```python
from build123d import *

# Parameters (mm, degrees)
SKETCH1_W           = 10.000000000000004
SKETCH1_H           = 10
SKETCH1_W_2         = 10
BOSS_EXTRUDE1_DEPTH = 60
CHAMFER1_SIZE       = 3
SKETCH2_R           = 2.5
BOSS_EXTRUDE2_DEPTH = 5
BOSS_EXTRUDE3_START = -65
SKETCH2_2_R         = 2.5
BOSS_EXTRUDE3_DEPTH = 5
CHAMFER2_SIZE       = 1
CHAMFER2_SIZE2      = 1.6731571851015
CHAMFER3_SIZE       = 0.75


with BuildPart() as part:
    # Sketch1 → Boss-Extrude1 (new body)
    with BuildSketch(Plane.XY):
        with Locations((-27.101007166283644, 56.98463103929536)):
            Rectangle(SKETCH1_W, SKETCH1_H)
        Polygon((-12.10100716628364, 51.98463103929536), (-15.740709508945711, 61.98463103929536), (-22.10100716628364, 61.98463103929536), (-22.10100716628364, 51.98463103929536), (-5, 5), (5, 5), align=None)
        Rectangle(SKETCH1_W_2, SKETCH1_H)
    extrude(amount=BOSS_EXTRUDE1_DEPTH)

    # Chamfer1
    chamfer1_edges = [part.edges().sort_by_distance(p)[0] for p in [
        (-5, -5, 30),
    ]]
    chamfer(chamfer1_edges, length=CHAMFER1_SIZE)

    # Sketch2 → Boss-Extrude2 (add)
    with BuildSketch(Plane.XY.offset(60)):
        Circle(SKETCH2_R)
    extrude(amount=BOSS_EXTRUDE2_DEPTH)

    # Sketch2<2> → Boss-Extrude3 (add)
    with BuildSketch(Plane.XY.offset(60).offset(BOSS_EXTRUDE3_START)):
        Circle(SKETCH2_2_R)
    extrude(amount=BOSS_EXTRUDE3_DEPTH)

    # Chamfer2
    chamfer2_edges = [part.edges().sort_by_distance(p)[0] for p in [
        (-15.740709508945711, 61.98463103929536, 30),
    ]]
    chamfer2_side = [part.faces().sort_by_distance(p)[0] for p in [
        (-5.3703547544728565, 33.492315519647676, 30),
    ]]
    chamfer(chamfer2_edges, length=CHAMFER2_SIZE, length2=CHAMFER2_SIZE2, reference=chamfer2_side[0])

    # Chamfer3
    chamfer3_edges = [part.edges().sort_by_distance(p)[0] for p in [
        (-2.5, 3.1e-16, 65),
        (-2.5, 3.1e-16, -5),
    ]]
    chamfer(chamfer3_edges, length=CHAMFER3_SIZE)


solid = part.part
```
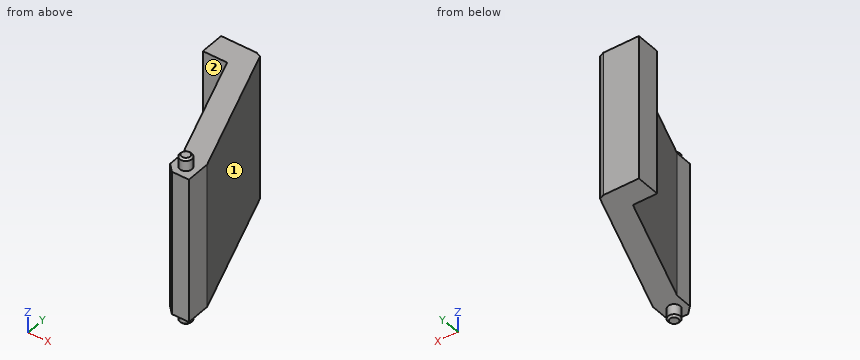
For this review, take the finished solid that the model builds, in its own axes (mm). Face numbers are marked on the shaded views. A direction names the side the tool comes from. Round coordinates to 2 decimals unless told otherwise and drop trailing zeros. Write each loop counter-clockwise with the first axis right and the second up, starting at its lowest first coordinate (ties: lowest second). Pieces come first, ordered by that corner, then holes. Notation, with made-up numbers: (27, 1) - (81, 1) arc R9 cw to (81, 15) - close; hole circle Ø3 at (31.5, 63.25). An arc over 180 degrees is marked (long way). Answer as CSV lines item,"result". Start each with the question number.
(1) Add section D-D, the plane x = -25. State the section outline as (y, z) points, plus the area to 3 significant figures.
(2) For line 1 (Y direction, x = -24, z = 32.5); line 2 (X direction, y = -1, z = 2.5); line 3 (Z direction, x = -7.5, y = 36), list the stretches that pass through material, from the lowest coordinate up.
(3) Machinability: for the marked faces 1 and 2, which of the approach directions +Z, -Z, +X, -X, +Y, -Y give a long, thin tool a straight path to every point of the face, cutting with its end or side? Answer none if there is none.
(4) For pin 1 (7.5 mm diameter, centred on y = 1.5, z = 24, fed in from -X); pin 2 (18.5 mm diameter, centred on x = -7, y = 30.5, fed in from -Z); pin 3 (3 mm diameter, centred on y = 33, z = 22.5, fed in from +X); pin 4 (5 mm diameter, centred on x = -11.5, y = 11.5, fed in from +Z), all flat-tipped, find the tip position at first contact; note any pin that passes through.
(5) Add section C-C, the plane x = 0. State the section outline as (y, z) points, plus the area to 3 significant figures.
(6) Add section B-B, the plane y = 0. State the section outline as (x, z) points, plus the area to 3 significant figures.
(7) Add section A-A, the plane z = 32. State the section outline as (x, y) points, plus the area to 3 significant figures.
From the geometry:
1,outline,"(51.98, 0) - (61.98, 0) - (61.98, 60) - (51.98, 60) - close"
1,area,"600 mm²"
2,line 1,"y = 51.98 to 61.98"
2,line 2,"x = -5 to 5"
2,line 3,"z = 0 to 60"
3,face 1,"+Z, -Z, +X, +Y"
3,face 2,"+Z, -Z, -X, -Y"
4,pin 1,"stops at x = -5.09"
4,pin 2,"stops at z = 0"
4,pin 3,"stops at x = -4.65"
4,pin 4,"passes through"
5,outline,"(-5, 0) - (-2.5, 0) - (-2.5, -4.25) - (-1.75, -5) - (1.75, -5) - (2.5, -4.25) - (2.5, 0) - (18.74, 0) - (18.74, 60) - (2.5, 60) - (2.5, 64.25) - (1.75, 65) - (-1.75, 65) - (-2.5, 64.25) - (-2.5, 60) - (-5, 60) - close"
5,area,"1,470 mm²"
6,outline,"(-5, 0) - (-2.5, 0) - (-2.5, -4.25) - (-1.75, -5) - (1.75, -5) - (2.5, -4.25) - (2.5, 0) - (5, 0) - (5, 60) - (2.5, 60) - (2.5, 64.25) - (1.75, 65) - (-1.75, 65) - (-2.5, 64.25) - (-2.5, 60) - (-5, 60) - close"
6,area,"649 mm²"
7,outline,"(-32.1, 51.98) - (-22.1, 51.98) - (-5, 5) - (-5, -2) - (-2, -5) - (5, -5) - (5, 5) - (-15.4, 61.04) - (-17.41, 61.98) - (-32.1, 61.98) - close"
7,area,"746 mm²"
